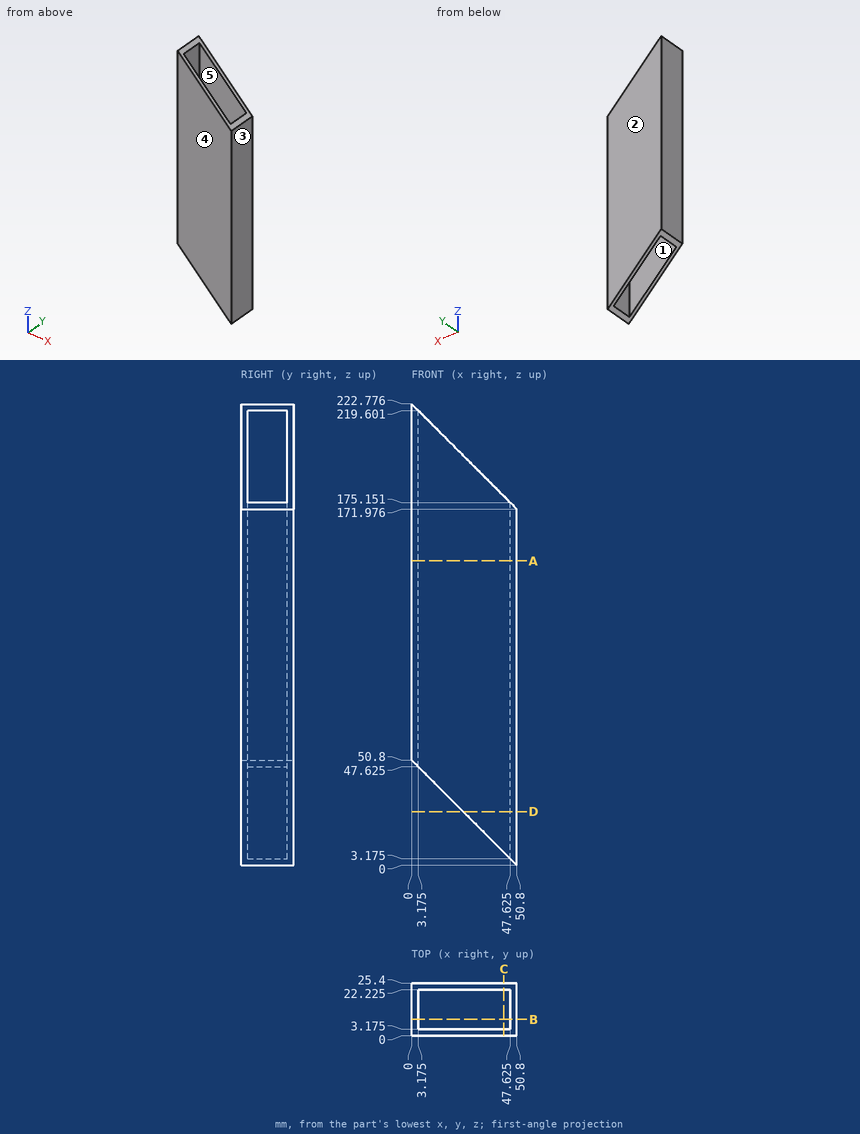
Could you check a few things on this drawing? It's one solid part, dimensions in mm from its lowest x, y, z. A direction names the side the tool comes from. Round coordinates to 2 decimals unless told otherwise and drop trailing zeros. Write each loop counter-clockwise with the first axis right and the second up, starting at its lowest first coordinate (ties: lowest second). Pieces come first, ordered by that corner, then holes. Notation, with made-up numbers: M -30,-10.5 L -14,-10.5 A30 ccw -14,27.5 Z; hole C -5,51.5 d8. An arc over 180 degrees is marked long. Answer as CSV lines item,"result". Start each with the question number.
1. Suppose I cut it at D-D on z = 26. Write out the boundary of the cut face in (x, y) (3 decimals).
2. Suppose I cut it at C-C on x = 44.5. Write out the boundary of the cut face in (y, z) (1 decimal), then the cut area to 3 significant figures.
3. On a 3-axis mill with a long thin cutter (end or side, diameter ignored), from which of +Z, -Z, +X, -X, +Y, -Y can I reach the whole of each face in a straight line? I mean the marked faces 1 and 2. Say none if no direction works.
4. Thinking about a two-plate mould opening in X: for the marked faces 3, 4 and 5, which applies, released by +X, released by -X, zero draft, split by the parting line, or undercut?
5. I need wall thicknesses on probe 1 along Y at (x, z) = (7, 94) (3 decimals); probe 2 along X at (y, z) = (16, 52.5) (3 decimals); probe 3 along X at (y, z) = (15, 13) (3 decimals). Which ranges of each line are inside material? Lowest first, please.
6. I'm going to push flat-ended pins straight in: pin 1 Ø12 at (x, y) = (42, 17) entering from +Z (1 decimal); pin 2 Ø10 at (x, y) = (42.5, 10) entering from -Z; pin 3 Ø2 at (x, y) = (10.5, 4) entering from +Z. Where does each tip first touch, or does it pass through?
7. Suppose I cut it at B-B on y = 8. Write out the boundary of the cut face in (x, z) (1 decimal), then the cut area to 3 significant figures.
8. Suppose I cut it at A-A on z = 147. Write out the boundary of the cut face in (x, y) (3 decimals).
Check result:
1,outline,"M 24.8,0 L 50.8,0 L 50.8,25.4 L 24.8,25.4 L 24.8,22.225 L 47.625,22.225 L 47.625,3.175 L 24.8,3.175 Z"
2,outline,"M 0,6.3 L 3.2,6.3 L 3.2,178.3 L 0,178.3 Z; M 22.2,6.3 L 25.4,6.3 L 25.4,178.3 L 22.2,178.3 Z"
2,area,"1,090 mm2"
3,face 1,"+Z, -Z"
3,face 2,"+Z, -Z, +X, -X, +Y"
4,face 3,"released by +X"
4,face 4,"zero draft"
4,face 5,"undercut"
5,probe 1,"y = 0 to 3.175, 22.225 to 25.4"
5,probe 2,"x = 0 to 3.175, 47.625 to 50.8"
5,probe 3,"x = 47.625 to 50.8"
6,pin 1,"stops at z = 183.7"
6,pin 2,"passes through"
6,pin 3,"stops at z = 212.84"
7,outline,"M 0,50.8 L 3.2,47.6 L 3.2,219.6 L 0,222.8 Z; M 47.6,3.2 L 50.8,0 L 50.8,172 L 47.6,175.2 Z"
7,area,"1,090 mm2"
8,outline,"M 0,0 L 50.8,0 L 50.8,25.4 L 0,25.4 Z; hole M 3.175,3.175 L 47.625,3.175 L 47.625,22.225 L 3.175,22.225 Z"
